CAD build for the part. Positions are in the model's coordinates, mm. Face numbers are marked on the shaded views. Give positions to 0.01 mm unless a question says otherwise; leave off trailing zeros. Loops run counter-clockwise (first coordinate to the right, second up) from the corner with the lowest first, then second, coordinate; pieces in that order, holes last.
Item 1: Saw through at C-C on z = 1.25. Give the cut face in (x, y), plus the area to 3 significant figures.
Item 2: Mould opens along Y. For the marked faces 1 and 2 say: released by +Y, released by -Y, zero draft, split by the parting line, or undercut.
Item 3: Probe probe 1 along Y at (x, z) = (4.5, 1.5); probe 2 along X at (y, z) = (-23.5, 1.5); probe 3 along Y at (x, z) = (0, 7.65). List the from-to ranges inside material, lowest first.
Item 4: Saw through at B-B on x = 0. Give the cut face in (y, z), plus the area to 3 significant figures.
Item 5: Saw through at A-A on y = 30. Give the cut face in (x, z), plus the area to 3 significant figures.
Item 6: Saw through at D-D on y = -38. Give the cut face in (x, z), plus the area to 3 significant figures.
Item 7: Drop flat-ended pins along their axis: P1, Ø0.8, axis at x = -0.5, z = 7.5, coming from the +Y side; P2, Ø1.1, axis at y = 2, z = 7.5, coming from the -X side; P3, Ø1.1, axis at y = -0.5, z = 7.5, coming from the +X side; P4, Ø4, axis at y = -40.5, z = 4.5, coming from the +X side. Give the stop position or say it passes through.
from build123d import *

# Parameters (mm, degrees)
CROQUIS1_W              = 70
CROQUIS1_H              = 115
SALIENTE_EXTRUIR1_DEPTH = 8
CHAFL_N1_SIZE           = 4
VACIADO1_T              = -1
CROQUIS2_R              = 4
CROQUIS2_W              = 10
CROQUIS2_H              = 25
CORTAR_EXTRUIR1_DEPTH   = 68.788273322


with BuildPart() as part:
    # Croquis1 → Saliente-Extruir1 (new body)
    with BuildSketch(Plane.XY):
        Rectangle(CROQUIS1_W, CROQUIS1_H)
    extrude(amount=SALIENTE_EXTRUIR1_DEPTH)

    # Chaflán1
    chafl_n1_edges = [part.edges().sort_by_distance(p)[0] for p in [
        (-35, 0, 8),
        (0, -57.5, 8),
        (35, 0, 8),
        (0, 57.5, 8),
    ]]
    chamfer(chafl_n1_edges, length=CHAFL_N1_SIZE)

    # Vaciado1
    vaciado1_openings = [part.faces().sort_by_distance(p)[0] for p in [
        (0, 0, 0),
    ]]
    offset(amount=VACIADO1_T, openings=vaciado1_openings, kind=Kind.INTERSECTION)

    # Croquis2 → Cortar-Extruir1 (cut, through all)
    with BuildSketch(Plane.XY.offset(8)):
        with Locations((0, 30)):
            Circle(CROQUIS2_R)
        with Locations((0, -30)):
            Circle(CROQUIS2_R)
        Rectangle(CROQUIS2_W, CROQUIS2_H)
    extrude(amount=-CORTAR_EXTRUIR1_DEPTH, mode=Mode.SUBTRACT)


solid = part.part
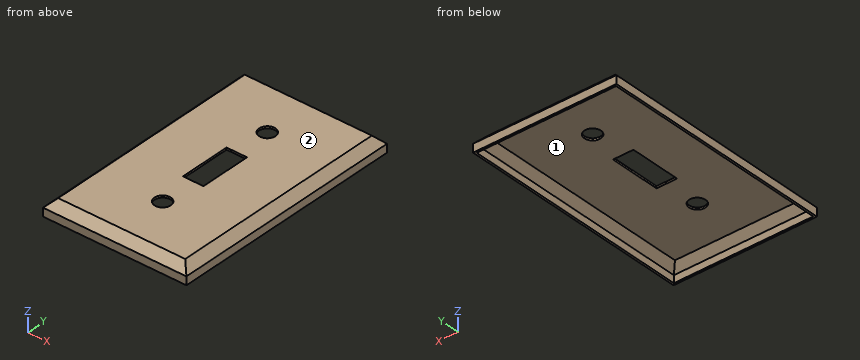
Results below:
1. outline: (-35, -57.5) - (35, -57.5) - (35, 57.5) - (-35, 57.5) - close; hole (-34, -56.5) - (34, -56.5) - (34, 56.5) - (-34, 56.5) - close
1. area: 366 mm2
2. face 1: undercut
2. face 2: zero draft
3. probe 1: y = -57.5 to -56.5, 56.5 to 57.5
3. probe 2: x = -35 to -34, 34 to 35
3. probe 3: y = -53.85 to -34, -26 to -12.5, 12.5 to 26, 34 to 53.85
4. outline: (-57.5, 0) - (-56.5, 0) - (-56.5, 3.59) - (-53.09, 7) - (-34, 7) - (-34, 8) - (-53.5, 8) - (-57.5, 4) - close; (-26, 7) - (-12.5, 7) - (-12.5, 8) - (-26, 8) - close; (12.5, 7) - (26, 7) - (26, 8) - (12.5, 8) - close; (34, 7) - (53.09, 7) - (56.5, 3.59) - (56.5, 0) - (57.5, 0) - (57.5, 4) - (53.5, 8) - (34, 8) - close
4. area: 83.7 mm2
5. outline: (-35, 0) - (-34, 0) - (-34, 3.59) - (-30.59, 7) - (-4, 7) - (-4, 8) - (-31, 8) - (-35, 4) - close; (4, 7) - (30.59, 7) - (34, 3.59) - (34, 0) - (35, 0) - (35, 4) - (31, 8) - (4, 8) - close
5. area: 71.7 mm2
6. outline: (-35, 0) - (-34, 0) - (-34, 3.59) - (-30.59, 7) - (30.59, 7) - (34, 3.59) - (34, 0) - (35, 0) - (35, 4) - (31, 8) - (-31, 8) - (-35, 4) - close
6. area: 79.7 mm2
7. P1: stops at y = 54.4
7. P2: stops at x = -32.05
7. P3: stops at x = 32.05
7. P4: stops at x = 35
